Can you work these out from the model? Positions are in its coordinate system, mm. Face numbers are marked on the shaded views. A direction names the side the tool comes from. Give positions to 0.01 mm unless a question says otherwise; leave off trailing zeros. Write each loop counter-clockwise with the first axis right and the second up, starting at its lowest first coordinate (ties: lowest second). Pieces come first, ordered by that corner, then holes. Notation, with made-up numbers: (-26, 58.25) -> (20, 58.25) arc R14 ccw to (20, 81.25) -> close; hole circle Ø9 at (-37, -31). An arc over 180 degrees is marked (long way). One line per item, written item: value.
from build123d import *

# Parameters (mm, degrees)
F1_DEPTH = 63.5
F0_W     = 25.4
F0_H     = 19.0494729435
F2_DEPTH = 25.4
F3_DEPTH = 7.9375
F5_R     = 5.08


with BuildPart() as f1:
    # F0 (on Front) → F1 (new body, symmetric)
    with BuildSketch(Plane.XZ):
        Polygon((-41.275, -9.525), (41.275, -9.525), (41.275, 9.525), (22.225, 9.525), (-41.275, 9.525), align=None)
    extrude(amount=F1_DEPTH, both=True)

    # F0 (on Front) → F2 (join, symmetric)
    with BuildSketch(Plane.XZ):
        with BuildLine():
            Line((22.225, 9.525), (41.275, 9.525))
            Line((41.275, 9.525), (41.275, 27.0002))
            ThreePointArc((41.275, 27.0002), (45.9246798487, 38.2255201513), (57.15, 42.8752))
            Line((57.15, 42.8752), (60.325, 42.8752))
            Line((60.325, 42.8752), (60.325, 61.9246729435))
            Line((60.325, 61.9246729435), (57.3418713593, 61.9246729435))
            add(Edge.make_bspline(
                [(49.0812338438, 60.9803506429), (51.8498488653, 61.3134633904), (54.5982729036, 61.6187718243), (57.3418713593, 61.9246729435)],
                knots=[0.9234728765, 0.9234728765, 0.9234728765, 0.9234728765, 1, 1, 1, 1], degree=3))
            ThreePointArc((49.0812338438, 60.9803506429), (29.7496598287, 48.6560764195), (22.225, 27.0002))
            Line((22.225, 27.0002), (22.225, 9.525))
        make_face()
        with Locations((73.025, 52.3999364718)):
            Rectangle(F0_W, F0_H)
    extrude(amount=F2_DEPTH, both=True)

    # F0 (on Front) → F3 (join, symmetric)
    with BuildSketch(Plane.XZ):
        with BuildLine():
            add(Edge.make_bspline(
                [(-41.275, 9.525), (-35.6876151592, 19.084335553), (-23.5641065751, 39.7994014349), (17.4108050565, 56.5096118561), (40.0708590665, 59.8962451699), (49.0812338438, 60.9803506429)],
                knots=[0, 0, 0, 0, 0.3116488423, 0.6744176422, 0.9234728765, 0.9234728765, 0.9234728765, 0.9234728765], degree=3))
            Line((-41.275, 9.525), (22.225, 9.525))
            Line((22.225, 9.525), (22.225, 27.0002))
            ThreePointArc((22.225, 27.0002), (29.7496598287, 48.6560764195), (49.0812338438, 60.9803506429))
        make_face()
    extrude(amount=F3_DEPTH, both=True)

    # F0 (on Front) → F4 (revolve)
    with BuildSketch(Plane.XZ):
        Polygon((85.725, 61.9246729435), (85.725, 42.8752), (85.725, 38.1), (111.125, 38.1), (111.125, 66.675), (85.725, 66.675), align=None)
    revolve(axis=Axis((85.725, 0, 52.3875), (0, 0, -1)))

    # F5
    f5_edges = [f1.edges().sort_by_distance(p)[0] for p in [
        (41.275, -63.5, 0),
        (-41.275, -63.5, 0),
        (-41.275, 63.5, 0),
        (41.275, 63.5, 0),
    ]]
    fillet(f5_edges, radius=F5_R)


solid = f1.part
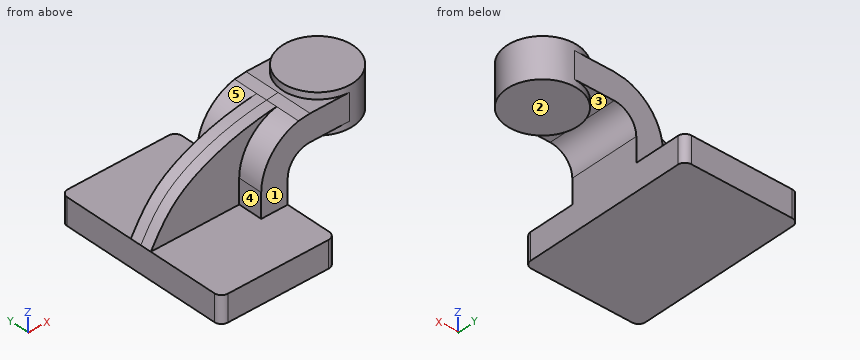
1) If we section it at C-C (y = 44.5): Write out the boundary of the cut face in (x, z) (3 decimals).
Answer list:
outline: (-41.275, -9.525) -> (41.275, -9.525) -> (41.275, 9.525) -> (-41.275, 9.525) -> close
2) If we section it at A-A (z = 6): Write out the boundary of the cut face in (x, y) (3 decimals), and give its area (3 significant figures).
Answer list:
outline: (-41.275, -58.42) arc R5.08 ccw to (-36.195, -63.5) -> (36.195, -63.5) arc R5.08 ccw to (41.275, -58.42) -> (41.275, 58.42) arc R5.08 ccw to (36.195, 63.5) -> (-36.195, 63.5) arc R5.08 ccw to (-41.275, 58.42) -> close
area: 10,500 mm^2
3) If we section it at B-B (x = 78.5): Write out the boundary of the cut face in (y, z) (3 decimals), and give its area (3 significant figures).
Answer list:
outline: (-25.4, 42.875) -> (-24.351, 42.875) -> (-24.351, 38.1) -> (24.351, 38.1) -> (24.351, 42.875) -> (25.4, 42.875) -> (25.4, 61.925) -> (24.351, 61.925) -> (24.351, 66.675) -> (-24.351, 66.675) -> (-24.351, 61.925) -> (-25.4, 61.925) -> close
area: 1,430 mm^2
4) Will these pins go through, and if not, where does the flat tip stop? pin 1 (10 mm diameter, centred on x = -13.5, y = 13, fed in from +Z) (3 decimals); pin 2 (5 mm diameter, centred on y = -17, z = 21.5, fed in from -X) (3 decimals); pin 3 (2 mm diameter, centred on x = 56.5, y = -4.5, fed in from +Z).
Answer list:
pin 1: stops at z = 9.525
pin 2: stops at x = 22.225
pin 3: stops at z = 61.92
5) I need wall thicknesses on L1, parallel to Y at x = 27, z = 23.5; L2, parallel to Z at x = -8, y = 41.5 (3 decimals); L3, parallel to X at y = -39, z = 8 (3 decimals). Which ranges of each line are inside material? Lowest first, please.
Answer list:
L1: y = -25.4 to 25.4
L2: z = -9.525 to 9.525
L3: x = -41.275 to 41.275
6) For the marked faces 1, 2, 3, 4 and 5, which set-ups out of +Z, -Z, +X, -X, +Y, -Y let a thin tool reach every point of the face, with its end or its side?
Answer list:
face 1: +Z, +X, -X, -Y
face 2: -Z, +X, +Y, -Y
face 3: -Z
face 4: +Z, -X, -Y
face 5: +Z, -X, +Y
